```python
from build123d import *

# Parameters (mm, degrees)
BOSS_EXTRUDE1_DEPTH = 38
SKETCH2_W           = 24.63
SKETCH2_H           = 45.13
CUT_EXTRUDE1_DEPTH  = 35
SKETCH3_W           = 24.63
SKETCH3_H           = 15.13
CUT_EXTRUDE2_DEPTH  = 35
FILLET1_R           = 1
SKETCH4_R           = 10
BOSS_EXTRUDE2_DEPTH = 1
FILLET3_R           = 1
SKETCH5_R           = 1.5
SKETCH5_R_2         = 4.5
CUT_EXTRUDE3_DEPTH  = 21
SKETCH6_W           = 24.981324159
SKETCH6_H           = 25
CUT_EXTRUDE4_DEPTH  = 35
FILLET2_R           = 1
FILLET4_R           = 1


with BuildPart() as part:
    # Sketch1 → Boss-Extrude1 (new body)
    with BuildSketch(Plane.XY):
        with BuildLine():
            Line((-72.469248292, 42.423690205), (1.530751708, 42.423690205))
            Line((1.530751708, 42.423690205), (1.530751708, -17.576309795))
            Line((1.530751708, -17.576309795), (-82.469248292, -17.576309795))
            Line((-82.469248292, -17.576309795), (-82.469248292, 32.423690205))
            ThreePointArc((-82.469248292, 32.423690205), (-79.540316103, 39.494758017), (-72.469248292, 42.423690205))
        make_face()
    extrude(amount=BOSS_EXTRUDE1_DEPTH)

    # Sketch2 → Cut-Extrude1 (cut)
    with BuildSketch(Plane.XY.offset(38)):
        with Locations((-38.765572451, 10.488690205)):
            Rectangle(SKETCH2_W, SKETCH2_H)
    extrude(amount=-CUT_EXTRUDE1_DEPTH, mode=Mode.SUBTRACT)

    # Sketch3 → Cut-Extrude2 (cut)
    with BuildSketch(Plane.XY.offset(3)):
        with Locations((-38.765572451, 10.488690205)):
            Rectangle(SKETCH3_W, SKETCH3_H)
    extrude(amount=-CUT_EXTRUDE2_DEPTH, mode=Mode.SUBTRACT)

    # Fillet1
    fillet1_edges = [part.edges().sort_by_distance(p)[0] for p in [
        (-79.540316103, 39.494758017, 38),
        (-82.469248292, 7.423690205, 38),
        (-51.080572451, 10.488690205, 38),
        (-40.469248292, -17.576309795, 38),
        (-38.765572451, -12.076309795, 38),
        (-26.450572451, 10.488690205, 38),
        (-38.765572451, 33.053690205, 38),
        (-38.765572451, 2.923690205, 0),
        (-26.450572451, 10.488690205, 0),
        (-38.765572451, 18.053690205, 0),
        (-51.080572451, 10.488690205, 0),
        (1.530751708, 12.423690205, 38),
        (-40.469248292, -17.576309795, 0),
        (-82.469248292, 7.423690205, 0),
        (-79.540316103, 39.494758017, 0),
        (-35.469248292, 42.423690205, 0),
        (1.530751708, 12.423690205, 0),
        (-35.469248292, 42.423690205, 38),
        (1.530751708, -17.576309795, 19),
        (-82.469248292, -17.576309795, 19),
        (1.530751708, 42.423690205, 19),
    ]]
    fillet(fillet1_edges, radius=FILLET1_R)

    # Sketch4 → Boss-Extrude2 (add)
    with BuildSketch(Plane(origin=(1.530751708, 0, 0), x_dir=(0, 0, -1), z_dir=(1, 0, 0))):
        with Locations(Location((-19, 0.423690205, 0), (0, 0, 270))):
            Circle(SKETCH4_R)
    extrude(amount=BOSS_EXTRUDE2_DEPTH)

    # Fillet3
    fillet3_edges = [part.edges().sort_by_distance(p)[0] for p in [
        (1.530751708, 10.423690205, 19),
    ]]
    fillet(fillet3_edges, radius=FILLET3_R - 0.0001)  # a hair under: the kernel refuses the full size

    # Sketch5 → Cut-Extrude3 (cut)
    with BuildSketch(Plane(origin=(2.530751708, 0, 0), x_dir=(0, 0, -1), z_dir=(1, 0, 0))):
        with Locations(Location((-19, 7.423690205, 0), (0, 0, 90))):
            Circle(SKETCH5_R)
        with Locations(Location((-12, 0.423690205, 0), (0, 0, 90))):
            Circle(SKETCH5_R)
        with Locations(Location((-19, -6.576309795, 0), (0, 0, 90))):
            Circle(SKETCH5_R)
        with Locations(Location((-26, 0.423690205, 0), (0, 0, 90))):
            Circle(SKETCH5_R)
        with Locations(Location((-19, 0.423690205, 0), (0, 0, 90))):
            Circle(SKETCH5_R_2)
    extrude(amount=-CUT_EXTRUDE3_DEPTH, mode=Mode.SUBTRACT)

    # Sketch6 → Cut-Extrude4 (cut)
    with BuildSketch(Plane.XY.offset(38)):
        with Locations((-13.959910372, 0.423690205)):
            Rectangle(SKETCH6_W, SKETCH6_H)
    extrude(amount=-CUT_EXTRUDE4_DEPTH, mode=Mode.SUBTRACT)

    # Fillet2
    fillet2_edges = [part.edges().sort_by_distance(p)[0] for p in [
        (-38.765572451, 2.923690205, 3),
        (-38.765572451, 18.053690205, 3),
    ]]
    fillet(fillet2_edges, radius=FILLET2_R)

    # Fillet4
    fillet4_edges = [part.edges().sort_by_distance(p)[0] for p in [
        (-26.450572451, 12.923690205, 20),
        (-26.157679232, 12.923690205, 37.707106781),
        (-26.450572451, 7.423690205, 3),
        (-13.459910371, 12.923690205, 38),
        (-13.459910371, -12.076309795, 38),
        (-1.469248292, 0.423690205, 38),
    ]]
    fillet(fillet4_edges, radius=FILLET4_R - 0.0001)  # a hair under: the kernel refuses the full size


solid = part.part
```
Input: part model. Units: mm. Frame: model coordinates. A direction names the side the tool comes from. Coordinates: 2 decimals unless noted, no trailing zeros. Loops run counter-clockwise (first coordinate to the right, second up) from the corner with the lowest first, then second, coordinate; pieces in that order, holes last.
Q1. Set-up query: faces 4 (the cylindrical face through (0.56, -0.16, 23.46)), 5 (the flat face through (2.531, -4, 21)), 6 (the flat face through (-26.451, 24, 19)). Return all of +Z, -Z, +X, -X, +Y, -Y with unobstructed straight access to the full face (end or side cutting, diameter ignored); none if empty.
Results are:
face 4: +X
face 5: +Z, -Z, +X, +Y, -Y
face 6: +Z
Q2. Contact query for flat-ended pins moving along their axis: pin 1 (18 mm diameter, centred on y = 23, z = 21, fed in from +X); pin 2 (7.5 mm diameter, centred on x = -36, y = -5, fed in from +Z). Output: stop coordinate, or through.
Results are:
pin 1: stops at x = 1.53
pin 2: stops at z = 3
Q3. Section A-A, the plane x = -33.5. Return the cut outline in (y, z).
Results are:
outline: (-17.58, 1) arc R1 ccw to (-16.58, 0) - (1.92, 0) arc R1 ccw to (2.92, 1) - (2.92, 2) arc R1 ccw to (1.92, 3) - (-12.08, 3) - (-12.08, 37) arc R1 ccw to (-13.08, 38) - (-16.58, 38) arc R1 ccw to (-17.58, 37) - close; (18.05, 1) arc R1 ccw to (19.05, 0) - (41.42, 0) arc R1 ccw to (42.42, 1) - (42.42, 37) arc R1 ccw to (41.42, 38) - (34.05, 38) arc R1 ccw to (33.05, 37) - (33.05, 3) - (19.05, 3) arc R1 ccw to (18.05, 2) - close
Q4. Section B-B, the plane z = 19. Give the number of separate pieces and of enclosed holes in the cut face, and give its area (3 significant figures).
Results are:
separate pieces: 3
enclosed holes: 0
area: 3,240 mm2
Q5. Line query: line 1 along X through (y, z) = (21, 19); line 2 along X through (y, z) = (2, 32.5); line 3 along Y through (x, z) = (-26.5, 14). Output: solid intervals per line, ascending.
Results are:
line 1: x = -82.47 to -51.08, -26.45 to 1.53
line 2: x = -82.47 to -51.08, -1.47 to 1.53
line 3: y = -17.58 to -12.08, 33.05 to 42.42
Q6. Section D-D, the plane z = 33. Return the cut outline in (x, y), and give its area (3 significant figures).
Results are:
outline: (-82.47, -16.58) arc R1 ccw to (-81.47, -17.58) - (0.53, -17.58) arc R1 ccw to (1.53, -16.58) - (1.53, 41.42) arc R1 ccw to (0.53, 42.42) - (-72.47, 42.42) arc R10 ccw to (-82.47, 32.42) - close; hole (-51.08, -12.08) - (-1.47, -12.08) - (-1.47, 12.92) - (-25.45, 12.92) arc R1 cw to (-26.45, 13.92) - (-26.45, 33.05) - (-51.08, 33.05) - close
area: 3,280 mm2
Q7. Section C-C, the plane x = -22.5. Return the cut outline in (y, z).
Results are:
outline: (-17.58, 1) arc R1 ccw to (-16.58, 0) - (41.42, 0) arc R1 ccw to (42.42, 1) - (42.42, 37) arc R1 ccw to (41.42, 38) - (13.92, 38) arc R1 ccw to (12.92, 37) - (12.92, 3) - (-12.08, 3) - (-12.08, 37) arc R1 ccw to (-13.08, 38) - (-16.58, 38) arc R1 ccw to (-17.58, 37) - close
Q8. Mould query, pull axis X, two halves, no side actions, for faces 1 (the flat face through (-27, -12.076, 20)), 2 (the cylindrical face through (0.559, -7.682, 20.014)), 3 (the flat face through (-82.469, 8, 19)). Classes: +X half, -X half, draft (parallel to the pull), parting line (faces both ways), or undercut.
Results are:
face 1: undercut
face 2: draft
face 3: -X half
